Design review of the part built by this model. Coordinates are the model's own, in mm. A direction names the side the tool comes from. Coordinates: 2 decimals unless noted, no trailing zeros. Loops run counter-clockwise (first coordinate to the right, second up) from the corner with the lowest first, then second, coordinate; pieces in that order, holes last. Notation, with made-up numbers: (30, 85) -> (55, 85) arc R24 cw to (55, 107) -> close; hole circle Ø7 at (20, 58.5). An arc over 180 degrees is marked (long way). Use one line per item in the form item = value. Start each with the question number.
1. Wall thickness on line 1 (Y direction, x = -11.6, z = 70); line 2 (X direction, y = 4.5, z = 84): over which ranges is each line inside the solid? List them lowest first. Write a range as from..to.
2. Consider section D-D (z = 57.5). State how many separate pieces and enclosed holes the cut face has, then the cut area to 3 significant figures.
3. Consider section B-B (y = 0). State the section outline as (x, z) points.
4. Consider section A-A (y = 11.6). State the section outline as (x, z) points.
5. Machinability: for faces 1 (the face through (-14, -4, 59)), 2 (the face through (14.43, 14.4, 60.84)), 3 (the face through (-14.43, 14.4, 60.84)), 4 (the face through (-6.444, 7.858, 59.16)), which of the approach directions +Z, -Z, +X, -X, +Y, -Y give a long, thin tool a straight path to every point of the face, cutting with its end or side? Answer none if there is none.
6. The part is to be moulded in two halves that separate along X. For faces 5 (the face through (9, -15, 59)), 6 (the face through (6.444, -7.858, 59.16)), 7 (the face through (15, -8, 59)), say which applies: released by +X, released by -X, zero draft, split by the parting line, or undercut.
7. For pin 1 (1.6 mm diameter, centred on y = 14, z = 62, fed in from -X); pin 2 (4.5 mm diameter, centred on x = 1, z = 84.5, fed in from +Y); pin 3 (1.6 mm diameter, centred on y = 14.5, z = 88.5, fed in from +X); pin 4 (3.5 mm diameter, centred on x = -11.6, y = 11.6, fed in from +Z), all flat-tipped, find the tip position at first contact; note any pin that passes through.
from build123d import *

# Parameters (mm, degrees)
SKETCH1_R           = 3.4
SKETCH1_R_2         = 2.1
BOSS_EXTRUDE1_DEPTH = 120
FILLET1_R           = 2


with BuildPart() as part:
    # Sketch1 → Boss-Extrude1 (new body)
    with BuildSketch(Plane.XY):
        Polygon((15, -15), (4, -15), (4, -13), (8.25, -13), (8.25, -9.664213562), (4.585786438, -6), (-4.585786438, -6), (-8.25, -9.664213562), (-8.25, -13), (-4, -13), (-4, -15), (-15, -15), (-15, -4), (-13, -4), (-13, -8.25), (-9.664213562, -8.25), (-6, -4.585786438), (-6, 4.585786438), (-9.664213562, 8.25), (-13, 8.25), (-13, 4), (-15, 4), (-15, 15), (-4, 15), (-4, 13), (-8.25, 13), (-8.25, 9.664213562), (-4.585786438, 6), (4.585786438, 6), (8.25, 9.664213562), (8.25, 13), (4, 13), (4, 15), (15, 15), (15, 4), (13, 4), (13, 8.25), (9.664213562, 8.25), (6, 4.585786438), (6, -4.585786438), (9.664213562, -8.25), (13, -8.25), (13, -4), (15, -4), align=None)
        Circle(SKETCH1_R, mode=Mode.SUBTRACT)
        with Locations((-11.6, 11.6)):
            Circle(SKETCH1_R_2, mode=Mode.SUBTRACT)
        with Locations((11.6, 11.6)):
            Circle(SKETCH1_R_2, mode=Mode.SUBTRACT)
        with Locations((11.6, -11.6)):
            Circle(SKETCH1_R_2, mode=Mode.SUBTRACT)
        with Locations((-11.6, -11.6)):
            Circle(SKETCH1_R_2, mode=Mode.SUBTRACT)
    extrude(amount=BOSS_EXTRUDE1_DEPTH)

    # Fillet1
    fillet1_edges = [part.edges().sort_by_distance(p)[0] for p in [
        (-15, -15, 60),
        (-15, 15, 60),
        (15, 15, 60),
        (15, -15, 60),
    ]]
    fillet(fillet1_edges, radius=FILLET1_R)


solid = part.part
Geometry check:
q1.line_1 = -15..-13.7, -9.5..-8.25, 8.25..9.5, 13.7..15
q1.line_2 = -15..-13, -6..6, 13..15
q2.separate_pieces = 1
q2.enclosed_holes = 5
q2.area = 333 mm²
q3.outline = (-6, 0) -> (-3.4, 0) -> (-3.4, 120) -> (-6, 120) -> close; (3.4, 0) -> (6, 0) -> (6, 120) -> (3.4, 120) -> close
q4.outline = (-15, 0) -> (-13.7, 0) -> (-13.7, 120) -> (-15, 120) -> close; (-9.5, 0) -> (-8.25, 0) -> (-8.25, 120) -> (-9.5, 120) -> close; (8.25, 0) -> (9.5, 0) -> (9.5, 120) -> (8.25, 120) -> close; (13.7, 0) -> (15, 0) -> (15, 120) -> (13.7, 120) -> close
q5.face_1 = +Z, -Z, -X
q5.face_2 = +Z, -Z, +X, +Y
q5.face_3 = +Z, -Z, -X, +Y
q5.face_4 = +Z, -Z
q6.face_5 = zero draft
q6.face_6 = undercut
q6.face_7 = released by +X
q7.pin_1 = -14.99
q7.pin_2 = 6
q7.pin_3 = 14.87
q7.pin_4 = through
